```python
from build123d import *

# Parameters (mm, degrees)
F0_W     = 25.4
F0_H     = 163.656833449
F0_W_2   = 136.525
F0_H_2   = 46.7590987682
F1_DEPTH = 19.05


with BuildPart() as f1:
    # F0 (on Front) → F1 (new body)
    with BuildSketch(Plane.XZ):
        with Locations((-79.4005683911, 253.7749098346)):
            Rectangle(F0_W, F0_H)
        Polygon((-66.7005683911, 171.9464931101), (-92.1005683911, 171.9464931101), (-92.1005683911, 146.5464931101), (-79.4005683911, 146.5464931101), (-79.4005683911, -12.6218702644), (-54.0005683911, -12.6218702644), (-54.0005683911, 108.4464931101), (142.8494316089, 108.4464931101), (142.8494316089, -107.4535068899), (180.9494316089, -107.4535068899), (180.9494316089, 171.9464931101), (180.9494316089, 288.8442277908), (44.4244316089, 288.8442277908), (44.4244316089, 335.6033265591), (-66.7005683911, 335.6033265591), align=None)
        with BuildLine():
            ThreePointArc((53.9494316089, 146.5464931101), (44.4244316089, 137.0214931101), (34.8994316089, 146.5464931101))
            ThreePointArc((34.8994316089, 146.5464931101), (44.4244316089, 156.0714931101), (53.9494316089, 146.5464931101))
        make_face(mode=Mode.SUBTRACT)
        Polygon((-79.4005683911, 146.5464931101), (-92.1005683911, 146.5464931101), (-92.1005683911, 121.1464931101), (-92.1005683911, -12.6218702644), (-79.4005683911, -12.6218702644), align=None)
        with BuildLine():
            Line((-92.1005683911, 451.3464931101), (-92.1005683911, 335.6033265591))
            Line((-92.1005683911, 335.6033265591), (-66.7005683911, 335.6033265591))
            Line((-66.7005683911, 335.6033265591), (44.4244316089, 335.6033265591))
            Line((44.4244316089, 335.6033265591), (180.9494316089, 335.6033265591))
            Line((180.9494316089, 335.6033265591), (180.9494316089, 451.3464931101))
            ThreePointArc((180.9494316089, 451.3464931101), (173.509943851, 469.3070053522), (155.5494316089, 476.7464931101))
            Line((155.5494316089, 476.7464931101), (-66.7005683911, 476.7464931101))
            ThreePointArc((-66.7005683911, 476.7464931101), (-84.6610806333, 469.3070053522), (-92.1005683911, 451.3464931101))
        make_face()
        with Locations((112.6869316089, 312.2237771749)):
            Rectangle(F0_W_2, F0_H_2)
        with BuildLine():
            Line((-79.4005683911, -12.6218702644), (-92.1005683911, -12.6218702644))
            Line((-92.1005683911, -12.6218702644), (-92.1005683911, -107.4535068899))
            ThreePointArc((-92.1005683911, -107.4535068899), (-88.6976136472, -120.1535068899), (-79.4005683911, -129.4505521461))
            Line((-79.4005683911, -129.4505521461), (-79.4005683911, -12.6218702644))
        make_face()
        with BuildLine():
            Line((-54.0005683911, -12.6218702644), (-79.4005683911, -12.6218702644))
            Line((-79.4005683911, -12.6218702644), (-79.4005683911, -129.4505521461))
            ThreePointArc((-79.4005683911, -129.4505521461), (-73.2745721367, -131.9880228777), (-66.7005683911, -132.8535068899))
            Line((-66.7005683911, -132.8535068899), (39.5014062524, -132.8535068899))
            Line((39.5014062524, -132.8535068899), (39.5014062524, -107.4535068899))
            Line((39.5014062524, -107.4535068899), (-54.0005683911, -107.4535068899))
            Line((-54.0005683911, -107.4535068899), (-54.0005683911, -12.6218702644))
        make_face()
        Polygon((39.5014062524, -107.4535068899), (39.5014062524, -132.8535068899), (104.7494316089, -132.8535068899), (104.7494316089, -107.4535068899), (95.2244316089, -107.4535068899), align=None)
        with BuildLine():
            ThreePointArc((155.5494316089, -132.8535068899), (173.509943851, -125.4140191321), (180.9494316089, -107.4535068899))
            Line((180.9494316089, -107.4535068899), (142.8494316089, -107.4535068899))
            Line((142.8494316089, -107.4535068899), (104.7494316089, -107.4535068899))
            Line((104.7494316089, -107.4535068899), (104.7494316089, -132.8535068899))
            Line((104.7494316089, -132.8535068899), (155.5494316089, -132.8535068899))
        make_face()
    extrude(amount=F1_DEPTH)


solid = f1.part
```
For this review, take the finished solid that the model builds, in its own axes (mm). A direction names the side the tool comes from. Round coordinates to 2 decimals unless told otherwise and drop trailing zeros. Write each loop counter-clockwise with the first axis right and the second up, starting at its lowest first coordinate (ties: lowest second). Pieces come first, ordered by that corner, then holes.
1) Take a section at B-B on x = -3. Give the boundary of the cut face in (y, z).
Answer below:
outline: (-19.05, -132.85) - (0, -132.85) - (0, -107.45) - (-19.05, -107.45) - close; (-19.05, 108.45) - (0, 108.45) - (0, 476.75) - (-19.05, 476.75) - close
2) For line 1 along Z through (x, y) = (-28, -4.5); line 2 along X through (y, z) = (-12, 99.5); line 3 along X through (y, z) = (-2.75, 145), list the stretches that pass through material, from the lowest coordinate up.
Answer below:
line 1: z = -132.85 to -107.45, 108.45 to 476.75
line 2: x = -92.1 to -54, 142.85 to 180.95
line 3: x = -92.1 to 35.03, 53.82 to 180.95
3) Mouldability with a two-part tool opening along Z and no side actions: class faces 3 (the face through (-54.001, -9, -1)), 4 (the face through (43, 0, 244)), 5 (the face through (43, -9, -132.854)), 6 (the face through (46.49, -9.39, 137.25)) as +Z half, -Z half, draft (parallel to the pull), parting line (faces both ways), or undercut.
Answer below:
face 3: undercut
face 4: draft
face 5: -Z half
face 6: undercut
4) Take a section at C-C on y = -12.25. State how many separate pieces and enclosed holes the cut face has, then the cut area to 3 significant figures.
Answer below:
separate pieces: 1
enclosed holes: 2
area: 123,000 mm2
5) Insertion check: pin 1 Ø11.5 at (x, z) = (44.42, 146.55) entering from +Y. The pin has a flat end and moves straight along its axis. Give the tip position at first contact, or say it passes through.
Answer below:
pin 1: passes through
6) Machinability: for faces 1 (the face through (43, -19.05, 244)), 2 (the face through (142.849, -9, 2)), which of the approach directions +Z, -Z, +X, -X, +Y, -Y give a long, thin tool a straight path to every point of the face, cutting with its end or side? Answer none if there is none.
Answer below:
face 1: +Z, -Z, +X, -X, -Y
face 2: +Y, -Y
7) Take a section at A-A on z = -71. Give the boundary of the cut face in (x, y), then the cut area to 3 significant figures.
Answer below:
outline: (-92.1, -19.05) - (-54, -19.05) - (-54, 0) - (-92.1, 0) - close; (142.85, -19.05) - (180.95, -19.05) - (180.95, 0) - (142.85, 0) - close
area: 1,450 mm2
